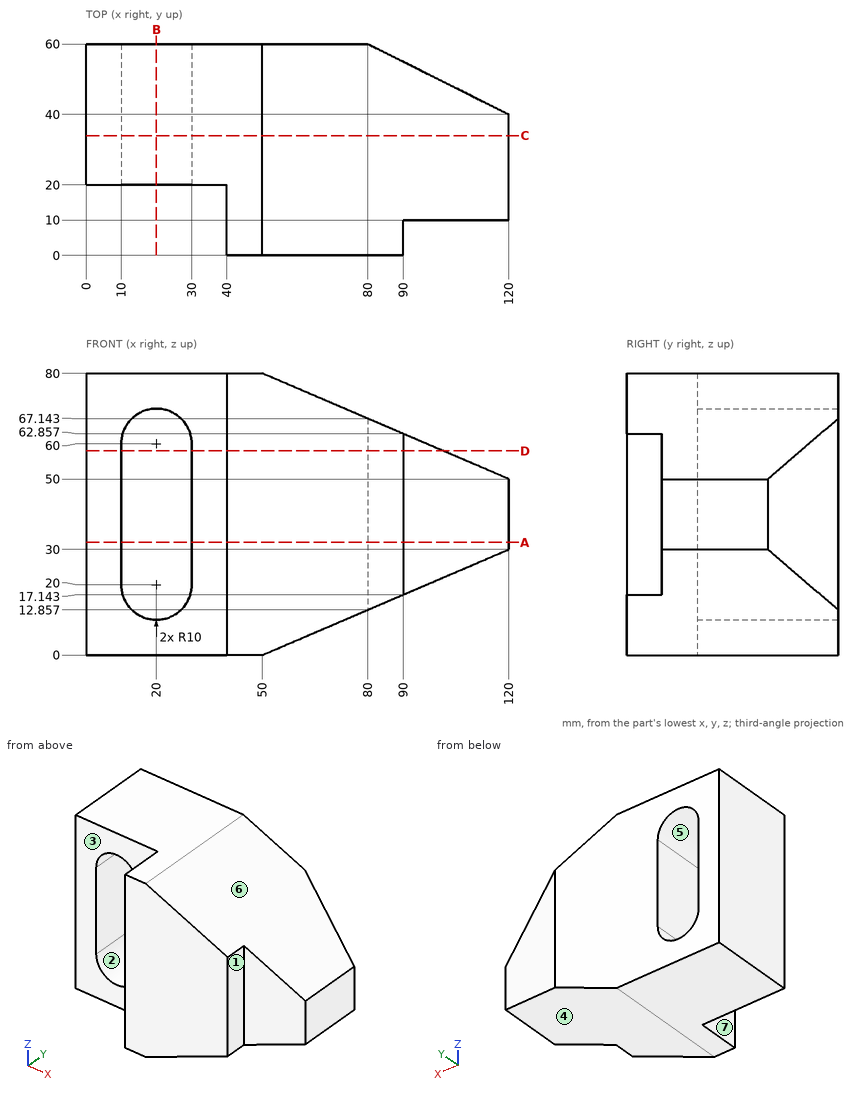
Check sheet for the drawn part. Datum: minimum x, y, z corner. Units: mm. A direction names the side the tool comes from. Coordinates: 2 decimals unless noted, no trailing zeros. Loops run counter-clockwise (first coordinate to the right, second up) from the corner with the lowest first, then second, coordinate; pieces in that order, holes last. Notation, with made-up numbers: (-10, 85.5) -> (6, 85.5) arc R28 ccw to (6, 113.5) -> close; hole circle Ø5 at (19, -7.5). An arc over 180 degrees is marked (long way). Answer as a JSON object with one key per item and string values. Group by question number.
Item 1: Sectioned sample at B-B on x = 20. Record the boundary of the cut face in (y, z).
Item 2: Scan lines: probe 1 along X at (y, z) = (55, 47); probe 2 along X at (y, z) = (11.5, 31.5); probe 3 along X at (y, z) = (45, 37). Record each from-to range of solid material in increasing order.
Item 3: Sectioned sample at A-A on z = 32. Record the boundary of the cut face in (x, y), plus the area to 3 significant figures.
Item 4: Sectioned sample at C-C on y = 34. Record the boundary of the cut face in (x, z), plus the area to 3 significant figures.
Item 5: Sectioned sample at D-D on z = 58. Record the boundary of the cut face in (x, y).
Item 6: Depth check by flat-ended pin: pin 1 (12 mm diameter, centred on y = 50, z = 36, fed in from +X); pin 2 (2 mm diameter, centred on x = 69, y = 40, fed in from -Z); pin 3 (8 mm diameter, centred on x = 104, z = 61.5, fed in from +Y); pin 4 (3 mm diameter, centred on x = 81.5, y = 51.5, fed in from -Z). Enter the tip coordinate at first touch or a pass-through.
Item 7: Mould release check, pull along Z, two halves, no side actions. Record for the marked faces 4, 5, 6 and 7: +Z half, -Z half, draft (parallel to the pull), parting line (faces both ways), or undercut.
Item 8: Tool access check on the marked faces 1, 2 and 3. Record the directions out of +Z, -Z, +X, -X, +Y, -Y that give a thin tool (end or side, any length) a straight path to the whole face; none if there is none.
Evaluation:
{
 "1": {"outline": "(20, 0) -> (60, 0) -> (60, 10) -> (20, 10) -> close; (20, 70) -> (60, 70) -> (60, 80) -> (20, 80) -> close"},
 "2": {"probe 1": "x = 0 to 10, 30 to 90", "probe 2": "x = 40 to 120", "probe 3": "x = 0 to 10, 30 to 110"},
 "3": {"outline": "(0, 20) -> (10, 20) -> (10, 60) -> (0, 60) -> close; (30, 20) -> (40, 20) -> (40, 0) -> (90, 0) -> (90, 10) -> (120, 10) -> (120, 40) -> (80, 60) -> (30, 60) -> close", "area": "4,900 mm²"},
 "4": {"outline": "(0, 0) -> (50, 0) -> (120, 30) -> (120, 50) -> (50, 80) -> (0, 80) -> close; hole (10, 20) arc R10 ccw to (30, 20) -> (30, 60) arc R10 ccw to (10, 60) -> close", "area": "6,390 mm²"},
 "5": {"outline": "(0, 20) -> (10, 20) -> (10, 60) -> (0, 60) -> close; (30, 20) -> (40, 20) -> (40, 0) -> (90, 0) -> (90, 10) -> (101.33, 10) -> (101.33, 49.33) -> (80, 60) -> (30, 60) -> close"},
 "6": {"pin 1": "stops at x = 112", "pin 2": "stops at z = 7.71", "pin 3": "passes through", "pin 4": "stops at z = 12.86"},
 "7": {"face 4": "-Z half", "face 5": "undercut", "face 6": "+Z half", "face 7": "draft"},
 "8": {"face 1": "+Z, -Z, +X, -Y", "face 2": "+Y, -Y", "face 3": "+Z, -Z, -X, -Y"}
}
